Check sheet for the modelled part. Datum: model origin and axes. Units: mm. Face numbers are marked on the shaded views. Give positions to 0.01 mm unless a question says otherwise; leave off trailing zeros. Order: outer loops, then holes, each group sorted by start corner. A loop starts at its lowest first (then second) coordinate and runs counter-clockwise, first axis right, second up.
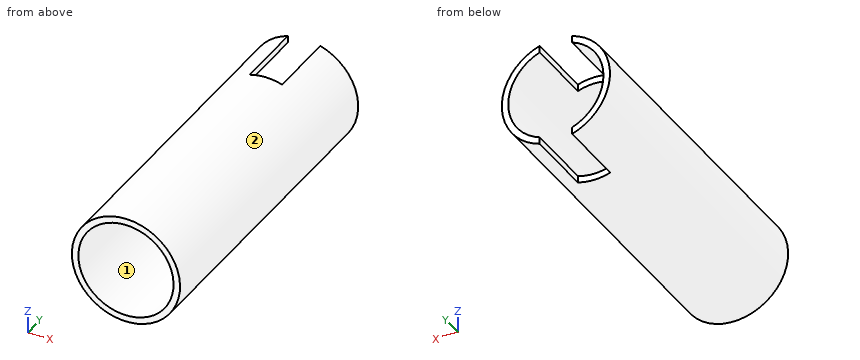
from build123d import *

# Parameters (mm, degrees)
ESBO_O1_R                = 25
ESBO_O1_R_2              = 22
RESSALTO_EXTRUS_O1_DEPTH = 150
CORTE_EXTRUS_O2_START    = -32.2
CORTE_EXTRUS_O2_DEPTH    = 32.2


with BuildPart() as part:
    # Esboço1 → Ressalto-extrusão1 (new body)
    with BuildSketch(Plane(origin=(0, 0, 0), x_dir=(1, 0, 0), z_dir=(0, 1, 0))):
        with Locations(Location((0, 0, 0), (0, 0, 270))):
            Circle(ESBO_O1_R)
        with Locations(Location((0, 0, 0), (0, 0, 270))):
            Circle(ESBO_O1_R_2, mode=Mode.SUBTRACT)
    extrude(amount=RESSALTO_EXTRUS_O1_DEPTH)

    # Esboço3 → Corte-extrusão2 (cut)
    with BuildSketch(Plane(origin=(0, 150, 0), x_dir=(1, 0, 0), z_dir=(0, 1, 0)).offset(CORTE_EXTRUS_O2_START)):
        with BuildLine():
            Line((7.5, -20.68211788), (7.5, -23.848480035))
            ThreePointArc((7.5, -23.848480035), (0, -25), (-7.5, -23.848480035))
            Line((-7.5, -23.848480035), (-7.5, -20.68211788))
            ThreePointArc((-7.5, -20.68211788), (0, -22), (7.5, -20.68211788))
        make_face()
        with BuildLine():
            Line((-7.5, 23.848480035), (-7.5, 20.68211788))
            ThreePointArc((-7.5, 20.68211788), (0, 22), (7.5, 20.68211788))
            Line((7.5, 20.68211788), (7.5, 23.848480035))
            ThreePointArc((7.5, 23.848480035), (0, 25), (-7.5, 23.848480035))
        make_face()
    extrude(amount=CORTE_EXTRUS_O2_DEPTH, mode=Mode.SUBTRACT)


solid = part.part
1) Section check A-A, the plane x = 0. Record the cut outline in (y, z).
Recorded:
outline: (0, -25) - (117.8, -25) - (117.8, -22) - (0, -22) - close; (0, 22) - (117.8, 22) - (117.8, 25) - (0, 25) - close
2) Material ranges on L1, parallel to X at y = 82.5, z = 1; L2, parallel to Z at x = 0, y = 106; L3, parallel to Z at x = -10, y = 42, recorded low to high.
Recorded:
L1: x = -24.98 to -21.98, 21.98 to 24.98
L2: z = -25 to -22, 22 to 25
L3: z = -22.91 to -19.6, 19.6 to 22.91
3) Section check C-C, the plane y = 43. Record the cut outline in (x, z), then the cut area to 3 significant figures.
Recorded:
outline: circle Ø50 at (0, 0); hole circle Ø44 at (0, 0)
area: 443 mm2
4) Section check B-B, the plane z = 0. Record the cut outline in (x, y).
Recorded:
outline: (-25, 0) - (-22, 0) - (-22, 150) - (-25, 150) - close; (22, 0) - (25, 0) - (25, 150) - (22, 150) - close
5) Draft check along Z on the marked faces 1 and 2. Enter one of: +Z half, -Z half, draft (parallel to the pull), parting line (faces both ways), or undercut.
Recorded:
face 1: undercut
face 2: parting line
6) Depth check by flat-ended pin: pin 1 Ø3.5 at (y, z) = (127, 21.5) entering from +X; pin 2 Ø10 at (x, z) = (-15, 0) entering from -Y; pin 3 Ø3.5 at (y, z) = (133, 22) entering from -X; pin 4 Ø2 at (x, y) = (2.5, 47.5) entering from -Z. Enter the tip coordinate at first touch or a pass-through.
Recorded:
pin 1: stops at x = 15.33
pin 2: passes through
pin 3: stops at x = -14.66
pin 4: stops at z = -24.95
